from build123d import *

# Parameters (mm, degrees)
BOSS_EXTRUDE1_DEPTH = 14.5
SKETCH2_W           = 26.5
SKETCH2_H           = 80
CUT_EXTRUDE1_DEPTH  = 15
SKETCH4_W           = 26.5
SKETCH4_H           = 14
CUT_EXTRUDE2_DEPTH  = 7
FILLET1_R           = 10
SKETCH5_W           = 3
SKETCH5_H           = 12
CUT_EXTRUDE3_DEPTH  = 29
CHAMFER1_SIZE       = 3
CHAMFER2_SIZE       = 2
BOSS_EXTRUDE2_DEPTH = 10
LPATTERN1_COUNT     = 17
LPATTERN1_PITCH     = 4.7
CUT_EXTRUDE4_DEPTH  = 76
SKETCH8_W           = 33.454520386
SKETCH8_H           = 107.037620526
CUT_EXTRUDE5_DEPTH  = 4.5
FILLET2_R           = 20
FILLET3_R           = 10
SKETCH9_W           = 25
SKETCH9_H           = 12.5
BOSS_EXTRUDE3_DEPTH = 22
FILLET4_R           = 5
SKETCH10_R          = 1.65
CUT_EXTRUDE6_DEPTH  = 22
SKETCH12_R          = 1.55
CUT_EXTRUDE7_DEPTH  = 22
CHAMFER3_SIZE       = 2
SKETCH13_W          = 23
SKETCH13_H          = 32
CUT_EXTRUDE8_DEPTH  = 3
FILLET5_R           = 5
SKETCH14_W          = 4
SKETCH14_H          = 10
BOSS_EXTRUDE4_DEPTH = 4.5
CHAMFER4_SIZE       = 2


with BuildPart() as part:
    # Sketch1 → Boss-Extrude1 (new body)
    with BuildSketch(Plane(origin=(0, 0, 0), x_dir=(1, 0, 0), z_dir=(0, 1, 0))):
        Polygon((-53.5, -24), (-39, 0), (0, 0), (0, -105), (-39, -105), (-53.5, -76), align=None)
    extrude(amount=BOSS_EXTRUDE1_DEPTH)

    # Sketch2 → Cut-Extrude1 (cut)
    with BuildSketch(Plane(origin=(0, 14.5, 0), x_dir=(1, 0, 0), z_dir=(0, 1, 0))):
        with Locations((-13.25, -65)):
            Rectangle(SKETCH2_W, SKETCH2_H)
    extrude(amount=-CUT_EXTRUDE1_DEPTH, mode=Mode.SUBTRACT)

    # Sketch4 → Cut-Extrude2 (cut)
    with BuildSketch(Plane.XZ):
        with Locations((-13.25, 18)):
            Rectangle(SKETCH4_W, SKETCH4_H)
    extrude(amount=-CUT_EXTRUDE2_DEPTH, mode=Mode.SUBTRACT)

    # Fillet1
    fillet1_edges = [part.edges().sort_by_distance(p)[0] for p in [
        (-26.5, 3.5, 11),
    ]]
    fillet(fillet1_edges, radius=FILLET1_R)

    # Sketch5 → Cut-Extrude3 (cut)
    with BuildSketch(Plane(origin=(0, 0, 0), x_dir=(-1, 0, 0), z_dir=(0, 0, -1))):
        with Locations((1.5, 6)):
            Rectangle(SKETCH5_W, SKETCH5_H)
    extrude(amount=-CUT_EXTRUDE3_DEPTH, mode=Mode.SUBTRACT)

    # Chamfer1
    chamfer1_edges = [part.edges().sort_by_distance(p)[0] for p in [
        (-3, 12, 12.5),
    ]]
    chamfer(chamfer1_edges, length=CHAMFER1_SIZE - 0.0001)  # a hair under: the kernel refuses the full size

    # Chamfer2
    chamfer2_edges = [part.edges().sort_by_distance(p)[0] for p in [
        (-14.75, 7, 25),
    ]]
    chamfer(chamfer2_edges, length=CHAMFER2_SIZE)

    # Sketch6 → Boss-Extrude2 (add)
    with BuildSketch(Plane.XZ):
        with BuildLine():
            Line((-26.5, 25.5), (-26.5, 22))
            Line((-26.5, 22), (-23.198291721, 23.283997664))
            ThreePointArc((-23.198291721, 23.283997664), (-22.879514851, 23.75), (-23.198291721, 24.216002336))
            Line((-23.198291721, 24.216002336), (-26.5, 25.5))
        make_face()
    boss_extrude2 = extrude(amount=-BOSS_EXTRUDE2_DEPTH)

    # LPattern1: Boss-Extrude2 ×17
    with Locations(*[(0, 0, i * LPATTERN1_PITCH) for i in range(1, LPATTERN1_COUNT)]):
        add(boss_extrude2)

    # Sketch7 → Cut-Extrude4 (cut)
    with BuildSketch(Plane.XY.offset(25)):
        Polygon((-26.5, 10), (-22.879514851, 7), (-22.879514851, 10), align=None)
    extrude(amount=CUT_EXTRUDE4_DEPTH, mode=Mode.SUBTRACT)

    # Sketch8 → Cut-Extrude5 (cut)
    with BuildSketch(Plane.XZ):
        with Locations((-47.227260193, 53.518810263)):
            Rectangle(SKETCH8_W, SKETCH8_H)
    extrude(amount=-CUT_EXTRUDE5_DEPTH, mode=Mode.SUBTRACT)

    # Fillet2
    fillet2_edges = [part.edges().sort_by_distance(p)[0] for p in [
        (-53.5, 9.5, 76),
        (-53.5, 9.5, 24),
    ]]
    fillet(fillet2_edges, radius=FILLET2_R)

    # Fillet3
    fillet3_edges = [part.edges().sort_by_distance(p)[0] for p in [
        (-39, 9.5, 105),
        (-39, 9.5, 0),
    ]]
    fillet(fillet3_edges, radius=FILLET3_R)

    # Sketch9 → Boss-Extrude3 (add)
    with BuildSketch(Plane(origin=(0, 14.5, 0), x_dir=(1, 0, 0), z_dir=(0, 1, 0))):
        with Locations((-12.5, -6.25)):
            Rectangle(SKETCH9_W, SKETCH9_H)
    extrude(amount=BOSS_EXTRUDE3_DEPTH)

    # Fillet4
    fillet4_edges = [part.edges().sort_by_distance(p)[0] for p in [
        (-25, 14.5, 6.25),
    ]]
    fillet(fillet4_edges, radius=FILLET4_R)

    # Sketch10 → Cut-Extrude6 (cut)
    with BuildSketch(Plane.XY.offset(12.5)):
        with Locations((-20, 31.5)):
            Circle(SKETCH10_R)
        with Locations((-5, 31.5)):
            Circle(SKETCH10_R)
        with Locations((-5, 19.5)):
            Circle(SKETCH10_R)
        with Locations((-20, 19.506382114)):
            Circle(SKETCH10_R)
    extrude(amount=-CUT_EXTRUDE6_DEPTH, mode=Mode.SUBTRACT)

    # Sketch12 → Cut-Extrude7 (cut)
    with BuildSketch(Plane(origin=(0, 14.5, 0), x_dir=(1, 0, 0), z_dir=(0, 1, 0))):
        with Locations(Location((-48, -48, 0), (0, 0, 270))):
            Circle(SKETCH12_R)
        with Locations(Location((-33, -48, 0), (0, 0, 270))):
            Circle(SKETCH12_R)
        with Locations(Location((-48, -58, 0), (0, 0, 270))):
            Circle(SKETCH12_R)
        with Locations(Location((-33, -58, 0), (0, 0, 270))):
            Circle(SKETCH12_R)
    extrude(amount=-CUT_EXTRUDE7_DEPTH, mode=Mode.SUBTRACT)

    # Chamfer3
    chamfer3_edges = [part.edges().sort_by_distance(p)[0] for p in [
        (-33, 14.5, 46.45),
        (-48, 14.5, 56.45),
        (-33, 14.5, 56.45),
        (-48, 14.5, 46.45),
    ]]
    chamfer(chamfer3_edges, length=CHAMFER3_SIZE)

    # Sketch13 → Cut-Extrude8 (cut)
    with BuildSketch(Plane.XZ.offset(-4.5)):
        with Locations((-42, 53)):
            Rectangle(SKETCH13_W, SKETCH13_H)
    extrude(amount=-CUT_EXTRUDE8_DEPTH, mode=Mode.SUBTRACT)

    # Fillet5
    fillet5_edges = [part.edges().sort_by_distance(p)[0] for p in [
        (-30.5, 2.25, 0),
    ]]
    fillet(fillet5_edges, radius=FILLET5_R)

    # Sketch14 → Boss-Extrude4 (add)
    with BuildSketch(Plane.XZ.offset(-4.5)):
        with Locations((-32.5, 25)):
            Rectangle(SKETCH14_W, SKETCH14_H)
    extrude(amount=BOSS_EXTRUDE4_DEPTH)

    # Chamfer4
    chamfer4_edges = [part.edges().sort_by_distance(p)[0] for p in [
        (-32.5, 0, 30),
    ]]
    chamfer(chamfer4_edges, length=CHAMFER4_SIZE)


solid = part.part
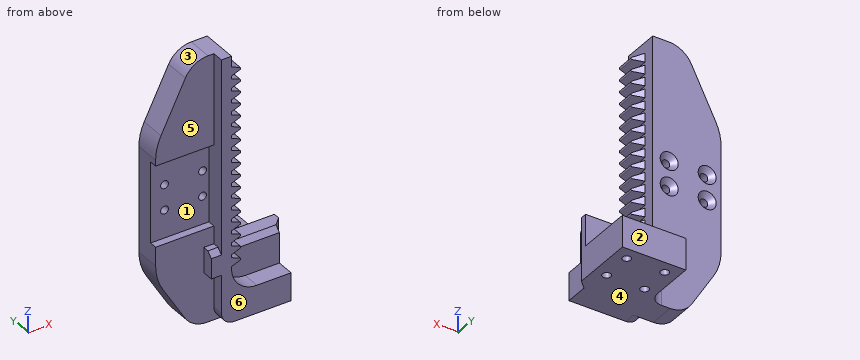
Could you check a few things on this model? Use its own coordinates, in mm. Face numbers are marked on the shaded views. A direction names the side the tool comes from. Coordinates: 2 decimals unless noted, no trailing zeros. Write each loop counter-clockwise with the first axis right and the second up, starting at its lowest first coordinate (ties: lowest second). Pieces come first, ordered by that corner, then holes. Notation, with made-up numbers: (47, 85.25) - (55, 85.25) arc R21 cw to (55, 123.25) - close; hole circle Ø5 at (35, 88.5). An arc over 180 degrees is marked (long way). Put each result on its own line as item: value. Start each with the question number.
Q1. Thinking about a two-plate mould opening in Z: for the marked faces 1, 2, 3 and 4, which applies, pulls with the +Z half, pulls with the -Z half, needs draft (parallel to the pull), parting line crosses it, or undercut?
Q2. I want a section at B-B on x = -48. Write out the boundary of the cut face in (y, z), plus the area to 3 significant figures.
Q3. Which directions (+Z, -Z, +X, -X, +Y, -Y) give clear straight access to the entire face, cutting with the end or side of a thin tool? Please do the marked faces 5 and 6.
Q4. I want a section at A-A on x = -20. Write out the boundary of the cut face in (y, z), plus the area to 3 significant figures.
Q5. Please list where these lines run through material, in increasing order: L1, parallel to Y at x = -20, z = 3.25; L2, parallel to Y at x = -5, z = 7; L3, parallel to X at y = 10.3, z = 58.
Q6. I'm going to push flat-ended pins straight in: P1, Ø3.5, axis at x = -33, z = 58, coming from the +Y side; P2, Ø5, axis at x = -31.5, z = 48.5, coming from the +Y side; P3, Ø3.5, axis at x = -37, y = 6.5, coming from the +Z side. Where does each tip first touch, or does it pass through?
Checks:
1. face 1: undercut
1. face 2: needs draft
1. face 3: pulls with the +Z half
1. face 4: pulls with the -Z half
2. outline: (4.5, 14.9) - (14.5, 14.9) - (14.5, 44.45) - (12.5, 46.45) - (7.5, 46.45) - (7.5, 37) - (4.5, 37) - close; (4.5, 69) - (7.5, 69) - (7.5, 59.55) - (12.5, 59.55) - (14.5, 61.55) - (14.5, 87) - (4.5, 87) - close; (7.5, 49.55) - (12.5, 49.55) - (14.5, 51.55) - (14.5, 54.45) - (12.5, 56.45) - (7.5, 56.45) - close
2. area: 574 mm²
3. face 5: +Z, -X, -Y
3. face 6: +Z, -Z, +X, -X, -Y
4. outline: (0, 0) - (17.86, 0) - (17.86, 12.5) - (14.5, 12.5) - (14.5, 25) - (9, 25) - (7, 23) - (7, 11.63) - (0, 11.63) - close; (21.16, 0) - (29.85, 0) - (29.85, 12.5) - (21.16, 12.5) - close; (33.15, 0) - (36.5, 0) - (36.5, 12.5) - (33.15, 12.5) - close
4. area: 459 mm²
5. L1: 0 to 17.86, 21.16 to 29.85, 33.15 to 36.5
5. L2: 0 to 17.85, 21.15 to 29.85, 33.15 to 36.5
5. L3: -53.5 to -49.55, -46.45 to -34.55, -31.45 to -26.5
6. P1: y = 12.7
6. P2: y = 14.5
6. P3: z = 104.7
